Could you check a few things on this model? Use its own coordinates, in mm. A direction names the side the tool comes from. Coordinates: 2 decimals unless noted, no trailing zeros. Loops run counter-clockwise (first coordinate to the right, second up) from the corner with the lowest first, then second, coordinate; pieces in that order, holes last. Notation, with made-up numbers: M 86.5,-29 L 145.5,-29 A19 cw 145.5,-16 Z; hole C -21,83.25 d9. An arc over 180 degrees is marked long. Write each question's results on one line, items separated by ' | '.
```python
from build123d import *

# Parameters (mm, degrees)
BOSS_EXTRUDE1_DEPTH = 78
BOSS_EXTRUDE2_START = 3
BOSS_EXTRUDE2_DEPTH = 3
CUT_EXTRUDE1_DEPTH  = 2
FILLET1_R           = 2
SKETCH5_R           = 2.25
CUT_EXTRUDE2_DEPTH  = 122.165176515
CHAMFER1_SIZE       = 1.5


with BuildPart() as part:
    # Sketch2 → Boss-Extrude1 (new body)
    with BuildSketch(Plane(origin=(0, 0, 0), x_dir=(1, 0, 0), z_dir=(0, 1, 0))):
        with BuildLine():
            Line((89, 0), (-89, 0))
            Line((-89, 0), (-89, -2))
            Line((-89, -2), (-63.5, -2))
            ThreePointArc((-63.5, -2), (-62.085786438, -2.585786438), (-61.5, -4))
            Line((-61.5, -4), (-61.5, -24))
            ThreePointArc((-61.5, -24), (-60.328427125, -26.828427125), (-57.5, -28))
            Line((-57.5, -28), (57.5, -28))
            ThreePointArc((57.5, -28), (60.328427125, -26.828427125), (61.5, -24))
            Line((61.5, -24), (61.5, -4))
            ThreePointArc((61.5, -4), (62.085786438, -2.585786438), (63.5, -2))
            Line((63.5, -2), (89, -2))
            Line((89, -2), (89, 0))
        make_face()
        with BuildLine():
            Line((57.5, -2), (-57.5, -2))
            ThreePointArc((-57.5, -2), (-58.914213562, -2.585786438), (-59.5, -4))
            Line((-59.5, -4), (-59.5, -24))
            ThreePointArc((-59.5, -24), (-58.914213562, -25.414213562), (-57.5, -26))
            Line((-57.5, -26), (57.5, -26))
            ThreePointArc((57.5, -26), (58.914213562, -25.414213562), (59.5, -24))
            Line((59.5, -24), (59.5, -4))
            ThreePointArc((59.5, -4), (58.914213562, -2.585786438), (57.5, -2))
        make_face(mode=Mode.SUBTRACT)
    extrude(amount=BOSS_EXTRUDE1_DEPTH)

    # Sketch3 → Boss-Extrude2 (add)
    with BuildSketch(Plane.XZ.offset(BOSS_EXTRUDE2_START)):
        with BuildLine():
            Line((-89, 2), (-89, 0))
            Line((-89, 0), (89, 0))
            Line((89, 0), (89, 2))
            Line((89, 2), (63.5, 2))
            ThreePointArc((63.5, 2), (62.085786438, 2.585786438), (61.5, 4))
            Line((61.5, 4), (61.5, 24))
            ThreePointArc((61.5, 24), (60.328427125, 26.828427125), (57.5, 28))
            Line((57.5, 28), (-57.5, 28))
            ThreePointArc((-57.5, 28), (-60.328427125, 26.828427125), (-61.5, 24))
            Line((-61.5, 24), (-61.5, 4))
            ThreePointArc((-61.5, 4), (-62.085786438, 2.585786438), (-63.5, 2))
            Line((-63.5, 2), (-89, 2))
        make_face()
    extrude(amount=-BOSS_EXTRUDE2_DEPTH)

    # Sketch4 → Cut-Extrude1 (cut)
    with BuildSketch(Plane.XY.offset(28)):
        with BuildLine():
            Line((-40, 24), (40, 24))
            ThreePointArc((40, 24), (42.828427125, 22.828427125), (44, 20))
            Line((44, 20), (44, 14))
            ThreePointArc((44, 14), (42.828427125, 11.171572875), (40, 10))
            Line((40, 10), (-40, 10))
            ThreePointArc((-40, 10), (-42.828427125, 11.171572875), (-44, 14))
            Line((-44, 14), (-44, 20))
            ThreePointArc((-44, 20), (-42.828427125, 22.828427125), (-40, 24))
        make_face()
    extrude(amount=-CUT_EXTRUDE1_DEPTH, mode=Mode.SUBTRACT)

    # Fillet1
    fillet1_edges = [part.edges().sort_by_distance(p)[0] for p in [
        (58.914213562, 0, 25.414213562),
        (59.5, 0, 14),
        (58.914213562, 0, 2.585786438),
        (0, 0, 2),
        (-58.914213562, 0, 2.585786438),
        (-59.5, 0, 14),
        (-58.914213562, 0, 25.414213562),
        (0, 0, 26),
    ]]
    fillet(fillet1_edges, radius=FILLET1_R)

    # Sketch5 → Cut-Extrude2 (cut, through all)
    with BuildSketch(Plane.XY.offset(2)):
        with Locations((-80, 70)):
            Circle(SKETCH5_R)
        with Locations((-80, 5)):
            Circle(SKETCH5_R)
        with Locations((80, 5)):
            Circle(SKETCH5_R)
        with Locations((80, 70)):
            Circle(SKETCH5_R)
    extrude(amount=-CUT_EXTRUDE2_DEPTH, mode=Mode.SUBTRACT)

    # Chamfer1
    chamfer1_edges = [part.edges().sort_by_distance(p)[0] for p in [
        (77.75, 70, 2),
        (77.75, 5, 2),
        (-82.25, 5, 2),
        (-82.25, 70, 2),
    ]]
    chamfer(chamfer1_edges, length=CHAMFER1_SIZE)


solid = part.part
```
(1) Imagine slicing it at C-C, the plane y = 70. State how many separate pieces and enclosed holes the cut face has, and give its area (3 significant figures).
Reported:
separate pieces: 3 | enclosed holes: 1 | area: 674 mm2
(2) Imagine slicing it at A-A, the plane y = 49. List the corners of the cut face in (x, z) for me, and give its area (3 significant figures).
Reported:
outline: M -89,0 L 89,0 L 89,2 L 63.5,2 A2 cw 61.5,4 L 61.5,24 A4 ccw 57.5,28 L -57.5,28 A4 ccw -61.5,24 L -61.5,4 A2 cw -63.5,2 L -89,2 Z; hole M -59.5,4 A2 ccw -57.5,2 L 57.5,2 A2 ccw 59.5,4 L 59.5,24 A2 ccw 57.5,26 L -57.5,26 A2 ccw -59.5,24 Z | area: 696 mm2
(3) Please list where these lines run through material, in increasing order: probe 1 along Y at (x, z) = (80, 0.1); probe 2 along X at (y, z) = (60.5, 20); probe 3 along Z at (x, y) = (8.5, 58.5). Write a range as from..to.
Reported:
probe 1: y = -3..2.75, 7.25..67.75, 72.25..78 | probe 2: x = -61.5..-59.5, 59.5..61.5 | probe 3: z = 0..2, 26..28
(4) Which directions (+Z, -Z, +X, -X, +Y, -Y) give clear straight access to the entire face, cutting with the end or side of a thin tool? Please do faces 5 (the cylindrical face through (-42.859, 22.797, 27.014)), 6 (the flat face through (59.5, 39, 14)), 7 (the flat face through (76, 37, 2)), 8 (the cylindrical face through (-60.297, 36.933, 26.859)), 9 (the cylindrical face through (-77.92, 4.14, 0.25)).
Reported:
face 5: +Z | face 6: +Y | face 7: +Z, +X, +Y, -Y | face 8: +Z, -X, +Y, -Y | face 9: +Z, -Z
(5) Will these pins go through, and if not, where does the flat tip stop? P1, Ø5, axis at y = 16, z = 6, coming from the +X side; P2, Ø1, axis at y = 17, z = 27, coming from the +X side; P3, Ø8, axis at y = 13, z = 11.5, coming from the +X side; P4, Ø2.5, axis at x = -80, y = 5, coming from the -Z side.
Reported:
P1: stops at x = 61.56 | P2: stops at x = 60.62 | P3: stops at x = 61.5 | P4: passes through
(6) Imagine slicing it at B-B, the plane x = 0. List the corners of the cut face in (y, z) for me, and give its area (3 significant figures).
Reported:
outline: M -3,0 L 78,0 L 78,2 L 2,2 A2 cw 0,4 L 0,24 A2 cw 2,26 L 10,26 L 10,28 L -3,28 Z; M 24,26 L 78,26 L 78,28 L 24,28 Z | area: 370 mm2
(7) Imagine slicing it at D-D, the plane z = 18. List the corners of the cut face in (x, y) for me.
Reported:
outline: M -61.5,-3 L 61.5,-3 L 61.5,78 L 59.5,78 L 59.5,2 A2 cw 57.5,0 L -57.5,0 A2 cw -59.5,2 L -59.5,78 L -61.5,78 Z
(8) If we mould it in two halves opening along X, with no side actions, what happens to faces 1 (the flat face through (61.5, 37, 14)), 2 (the flat face through (1, 39, 2)), 3 (the cylindrical face through (-77.92, 69.14, 0.25)), 4 (the flat face through (-76, 37, 2))? For each: released by +X, released by -X, zero draft, split by the parting line, or undercut.
Reported:
face 1: released by +X | face 2: undercut | face 3: undercut | face 4: zero draft
